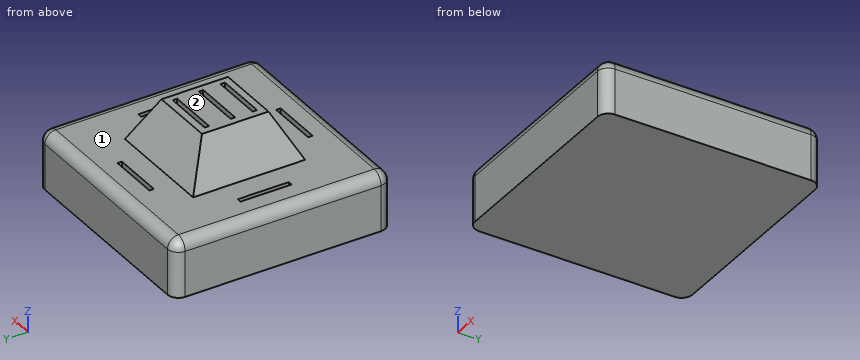
```python
from build123d import *

# Parameters (mm, degrees)
F0_W         = 101.6
F0_H         = 101.6
F1_DEPTH     = 50.8
F2_W         = 50.8819408715
F2_H         = 52.3191291059
F6_R         = 5.08
F7_T1_DEPTH  = 58.42
F7_S5_W      = 5.08
F7_S5_H      = 5.08
F7_T6_DEPTH  = 5.08
F7_S11_W     = 5.08
F7_S11_H     = 5.08
F7_T12_DEPTH = 5.08
F7_S17_W     = 5.08
F7_S17_H     = 5.08
F7_T18_DEPTH = 5.08
F7_S23_W     = 5.08
F7_S23_H     = 5.08
F7_T24_DEPTH = 5.08
F8_W         = 36.9938705117
F8_H         = 32.6922610402
F9_DEPTH     = 43.434
F10_W        = 2.0828
F10_H        = 23.876
F10_W_2      = 23.876
F10_H_2      = 2.0828
F11_DEPTH    = 15.748
F12_W        = 11.7269940674
F12_H        = 2.0828
F12_W_2      = 12.1490059326
F13_DEPTH    = 15.748
F14_DEPTH    = 24.384


# Not quite as in the source:
# - a fillet or chamfer that OpenCascade refuses, or shapes differently, is made with other operations: its cross-section is extruded or revolved along the edge and cut away or added


with BuildPart() as f1:
    # F0 (on Top) → F1 (new body)
    with BuildSketch(Plane.XY):
        with Locations((3.134034574, 24.3160160567)):
            Rectangle(F0_W, F0_H)
    extrude(amount=F1_DEPTH)

    # F2 (on face) → F5 section 0
    with BuildSketch(Plane.XY.offset(50.8), mode=Mode.PRIVATE) as f5_s0:
        with Locations((3.134034574, 24.3160160567)):
            Rectangle(F2_W, F2_H)
    loft([Vertex(3.134034574, 24.3160160567, 101.6), f5_s0.sketch])

    # F6
    f6_edges = [f1.edges().sort_by_distance(p)[0] for p in [
        (3.134035, -26.483984, 50.8),
        (-47.665965, 24.316016, 50.8),
        (3.134035, 75.116016, 50.8),
        (53.934035, 24.316016, 50.8),
    ]]
    fillet(f6_edges, radius=F6_R)

    # F7: fillet of radius 5.08 on 4 edges, made by hand

    # F7_s2 → F7_t1 (cut)
    with BuildSketch(Plane.XY.offset(-12.7)):
        with BuildLine():
            ThreePointArc((-42.585965426, 75.1160160567), (-46.1780678744, 73.6281185051), (-47.665965426, 70.0360160567))
            Line((-47.665965426, 70.0360160567), (-47.665965426, 75.1160160567))
            Line((-47.665965426, 75.1160160567), (-42.585965426, 75.1160160567))
        make_face()
        with BuildLine():
            ThreePointArc((-47.665965426, -21.4039839433), (-46.1780678744, -24.9960863917), (-42.585965426, -26.4839839433))
            Line((-42.585965426, -26.4839839433), (-47.665965426, -26.4839839433))
            Line((-47.665965426, -26.4839839433), (-47.665965426, -21.4039839433))
        make_face()
        with BuildLine():
            ThreePointArc((53.934034574, -21.4039839433), (52.4461370225, -24.9960863917), (48.854034574, -26.4839839433))
            Line((48.854034574, -26.4839839433), (53.934034574, -26.4839839433))
            Line((53.934034574, -26.4839839433), (53.934034574, -21.4039839433))
        make_face()
        with BuildLine():
            ThreePointArc((48.854034574, 75.1160160567), (52.4461370225, 73.6281185051), (53.934034574, 70.0360160567))
            Line((53.934034574, 70.0360160567), (53.934034574, 75.1160160567))
            Line((53.934034574, 75.1160160567), (48.854034574, 75.1160160567))
        make_face()
    extrude(amount=F7_T1_DEPTH, mode=Mode.SUBTRACT)


with BuildPart() as f7_tool4:
    # F7_s5 → F7_t6 (new body)
    with BuildSketch(Plane.XZ.offset(-70.0360160567)):
        with Locations((51.394034574, 48.26)):
            Rectangle(F7_S5_W, F7_S5_H)
    extrude(amount=-F7_T6_DEPTH)

    # F7_s7 → F7_t8 (revolve, cut)
    with BuildSketch(Plane(origin=(48.854034574, 70.0360160567, 45.72), x_dir=(-0.7071067812, 0, -0.7071067812), z_dir=(0.7071067812, 0, -0.7071067812))):
        with BuildLine():
            ThreePointArc((0, -5.08), (5.08, 0), (0, 5.08))
            Line((0, 5.08), (0, -5.08))
        make_face()
    revolve(axis=Axis((48.854034574, 70.0360160567, 45.72), (0, 1, 0)), mode=Mode.SUBTRACT)


with BuildPart() as f1_1:
    add(f1.part)

    # F7_t3: cut F7_tool4
    add(f7_tool4.part, mode=Mode.SUBTRACT)


with BuildPart() as f7_tool10:
    # F7_s11 → F7_t12 (new body)
    with BuildSketch(Plane.YZ.offset(48.854034574)):
        with Locations((-23.9439839433, 48.26)):
            Rectangle(F7_S11_W, F7_S11_H)
    extrude(amount=F7_T12_DEPTH)

    # F7_s13 → F7_t14 (revolve, cut)
    with BuildSketch(Plane(origin=(48.854034574, -21.4039839433, 45.72), x_dir=(0, 0.7071067812, -0.7071067812), z_dir=(0, -0.7071067812, -0.7071067812))):
        with BuildLine():
            ThreePointArc((0, -5.08), (5.08, 0), (0, 5.08))
            Line((0, 5.08), (0, -5.08))
        make_face()
    revolve(axis=Axis((48.854034574, -21.4039839433, 45.72), (1, 0, 0)), mode=Mode.SUBTRACT)


with BuildPart() as f1_2:
    add(f1_1.part)

    # F7_t9: cut F7_tool10
    add(f7_tool10.part, mode=Mode.SUBTRACT)


with BuildPart() as f7_tool16:
    # F7_s17 → F7_t18 (new body)
    with BuildSketch(Plane.YZ.offset(-42.585965426)):
        with Locations((-23.9439839433, 48.26)):
            Rectangle(F7_S17_W, F7_S17_H)
    extrude(amount=-F7_T18_DEPTH)

    # F7_s19 → F7_t20 (revolve, cut)
    with BuildSketch(Plane(origin=(-42.585965426, -21.4039839433, 45.72), x_dir=(0, 0.7071067812, -0.7071067812), z_dir=(0, 0.7071067812, 0.7071067812))):
        with BuildLine():
            ThreePointArc((0, -5.08), (5.08, 0), (0, 5.08))
            Line((0, 5.08), (0, -5.08))
        make_face()
    revolve(axis=Axis((-42.585965426, -21.4039839433, 45.72), (-1, 0, 0)), mode=Mode.SUBTRACT)


with BuildPart() as f1_3:
    add(f1_2.part)

    # F7_t15: cut F7_tool16
    add(f7_tool16.part, mode=Mode.SUBTRACT)


with BuildPart() as f7_tool22:
    # F7_s23 → F7_t24 (new body)
    with BuildSketch(Plane.XZ.offset(-70.0360160567)):
        with Locations((-45.125965426, 48.26)):
            Rectangle(F7_S23_W, F7_S23_H)
    extrude(amount=-F7_T24_DEPTH)

    # F7_s25 → F7_t26 (revolve, cut)
    with BuildSketch(Plane(origin=(-42.585965426, 70.0360160567, 45.72), x_dir=(0.7071067812, 0, -0.7071067812), z_dir=(0.7071067812, 0, 0.7071067812))):
        with BuildLine():
            ThreePointArc((0, -5.08), (5.08, 0), (0, 5.08))
            Line((0, 5.08), (0, -5.08))
        make_face()
    revolve(axis=Axis((-42.585965426, 70.0360160567, 45.72), (0, 1, 0)), mode=Mode.SUBTRACT)


with BuildPart() as f1_4:
    add(f1_3.part)

    # F7_t21: cut F7_tool22
    add(f7_tool22.part, mode=Mode.SUBTRACT)

    # F8 (on Front) → F9 (cut)
    with BuildSketch(Plane.XZ):
        with Locations((2.3658862337, 87.7631418407)):
            Rectangle(F8_W, F8_H)
    extrude(amount=-F9_DEPTH, mode=Mode.SUBTRACT)

    # F10 (on face) → F11 (cut)
    with BuildSketch(Plane.XY.offset(50.8)):
        with Locations((-33.924565426, 24.3160160567)):
            Rectangle(F10_W, F10_H)
        with Locations((3.134034574, 61.3746160567)):
            Rectangle(F10_W_2, F10_H_2)
        with Locations((40.192634574, 24.3160160567)):
            Rectangle(F10_W, F10_H)
        with Locations((3.134034574, -12.7425839433)):
            Rectangle(F10_W_2, F10_H_2)
    extrude(amount=-F11_DEPTH, mode=Mode.SUBTRACT)

    # F12 (on face) → F13 (cut)
    with BuildSketch(Plane.XY.offset(71.4170113206)):
        with Locations((-2.7294624597, 35.4132379736)):
            Rectangle(F12_W, F12_H)
        with Locations((9.2085375403, 35.4132379736)):
            Rectangle(F12_W_2, F12_H)
        with Locations((9.2085375403, 13.0715451534)):
            Rectangle(F12_W_2, F12_H)
        with Locations((-2.7294624597, 13.0715451534)):
            Rectangle(F12_W, F12_H)
        with Locations((-2.7294624597, 23.2746160567)):
            Rectangle(F12_W, F12_H)
        with Locations((9.2085375403, 23.2746160567)):
            Rectangle(F12_W_2, F12_H)
    extrude(amount=-F13_DEPTH, mode=Mode.SUBTRACT)

    # F0 (on Top) → F14 (cut)
    with BuildSketch(Plane.XY):
        with Locations((3.134034574, 24.3160160567)):
            Rectangle(F0_W, F0_H)
    extrude(amount=F14_DEPTH, mode=Mode.SUBTRACT)


solid = f1_4.part
```
Geometry: final body of the model. Coordinates: model frame, mm. Face numbers are marked on the shaded views. A direction names the side the tool comes from. Round coordinates to 2 decimals unless told otherwise and drop trailing zeros. Write each loop counter-clockwise with the first axis right and the second up, starting at its lowest first coordinate (ties: lowest second). Pieces come first, ordered by that corner, then holes. Notation, with made-up numbers: (73, 76.25) -> (88, 76.25) arc R29 cw to (88, 100.25) -> close; hole circle Ø3 at (45.5, 51.5). An arc over 180 degrees is marked (long way). Use CSV: the item, a comma, the result in double quotes. Start each with the question number.
Q1. Reachability of the marked faces 1 and 2 from +Z, -Z, +X, -X, +Y, -Y: full face, straight path, thin tool, end or side. Return the list, or none.
Q2. Line query: L1, parallel to X at y = 35.5, z = 42.5; L2, parallel to Y at x = 8, z = 38.5; L3, parallel to Z at x = -26, y = 27.5. Output: solid intervals per line, ascending.
Q3. Section D-D (z = 64). Return loops of the section in (x, y), plus the area to 3 significant figures.
Q4. Section A-A (z = 42.5). Return loops of the section in (x, y).
Q5. First-contact query: pin 1 Ø12 at (x, z) = (-29.5, 58.5) entering from -Y; pin 2 Ø1.7 at (x, y) = (-34, 29.5) entering from +Z; pin 3 Ø17.5 at (x, z) = (-0.5, 61.5) entering from -Y; pin 4 Ø1 at (y, z) = (23.5, 61.5) entering from +X. Flat tips, straight axial feed; report the tip coordinate or a pass-through.
Q6. Section C-C (y = 2). Return loops of the section in (x, z) (3 decimals).
Result sheet:
1,face 1,"+Z"
1,face 2,"+Z, +X, -X, +Y, -Y"
2,L1,"-47.67 to -34.97, -32.88 to 39.15, 41.23 to 53.93"
2,L2,"-26.48 to -13.78, -11.7 to 60.33, 62.42 to 75.12"
2,L3,"24.38 to 50.8"
3,outline,"(-15.7, 4.95) -> (21.96, 4.95) -> (21.96, 43.68) -> (-15.7, 43.68) -> close; hole (-8.59, 12.03) -> (15.28, 12.03) -> (15.28, 14.11) -> (-8.59, 14.11) -> close; hole (-8.59, 22.23) -> (15.28, 22.23) -> (15.28, 24.32) -> (-8.59, 24.32) -> close; hole (-8.59, 34.37) -> (15.28, 34.37) -> (15.28, 36.45) -> (-8.59, 36.45) -> close"
3,area,"1,310 mm²"
4,outline,"(-47.67, -21.4) arc R5.08 ccw to (-42.59, -26.48) -> (48.85, -26.48) arc R5.08 ccw to (53.93, -21.4) -> (53.93, 70.04) arc R5.08 ccw to (48.85, 75.12) -> (-42.59, 75.12) arc R5.08 ccw to (-47.67, 70.04) -> close; hole (-34.97, 12.38) -> (-32.88, 12.38) -> (-32.88, 36.25) -> (-34.97, 36.25) -> close; hole (-8.8, -13.78) -> (15.07, -13.78) -> (15.07, -11.7) -> (-8.8, -11.7) -> close; hole (-8.8, 60.33) -> (15.07, 60.33) -> (15.07, 62.42) -> (-8.8, 62.42) -> close; hole (39.15, 12.38) -> (41.23, 12.38) -> (41.23, 36.25) -> (39.15, 36.25) -> close"
5,pin 1,"through"
5,pin 2,"z = 35.05"
5,pin 3,"y = -0.84"
5,pin 4,"x = 23.47"
6,outline,"(-47.666, 24.384) -> (53.934, 24.384) -> (53.934, 45.72) arc R5.08 ccw to (48.854, 50.8) -> (28.575, 50.8) -> (24.837, 58.264) -> (-18.569, 58.264) -> (-22.307, 50.8) -> (-42.586, 50.8) arc R5.08 ccw to (-47.666, 45.72) -> close"
